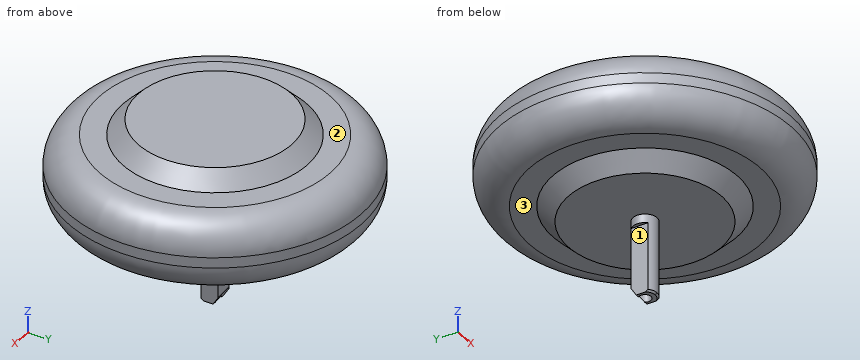
from build123d import *

# Parameters (mm, degrees)
SKETCH_1_R           = 85
EXTRUDE_1_DEPTH      = 21
SKETCH_2_R           = 54.5
EXTRUDE_2_DEPTH      = 30
CHAMFER_1_SIZE       = 10
SKETCH_3_R           = 7
EXTRUDE_3_DEPTH      = 45
SKETCH_5_OUTSIDE_W   = 224.47
SKETCH_5_OUTSIDE_H   = 224.47
SKETCH_5_OUTSIDE_W_2 = 9.85
SKETCH_5_OUTSIDE_H_2 = 14
CUT_EXTRUDE_1_DEPTH  = 40
CHAMFER_3_SIZE       = 1
SKETCH_7_R           = 3.5
CUT_EXTRUDE_2_DEPTH  = 45
FILLET_1_R           = 18
CUT_EXTRUDE_3_REACH  = 146.695


with BuildPart() as part:
    # 草图1 → 凸台-拉伸1 (new, symmetric)
    with BuildSketch(Plane.XY):
        with Locations(Location((0, 0, 0), (0, 0, 180))):
            Circle(SKETCH_1_R)
    extrude(amount=EXTRUDE_1_DEPTH, both=True)

    # 草图2 → 凸台-拉伸2 (add, symmetric)
    with BuildSketch(Plane.XY):
        Circle(SKETCH_2_R)
    extrude(amount=EXTRUDE_2_DEPTH, both=True)

    # 倒角1
    # the kernel refuses this chamfer: 10 mm, written as the material it takes off along each edge
    with BuildSketch(Plane(origin=(0, 0, -30), x_dir=(1, 0, 0), z_dir=(0, -1, 0))) as chamfer_1_piece_1_section:
        Polygon((54.5, CHAMFER_1_SIZE), (54.5 - CHAMFER_1_SIZE, 0), (54.5, 0), align=None)
    chamfer_1_piece_1 = revolve(axis=Axis((0, 0, -30), (0, 0, 1)), mode=Mode.PRIVATE)
    chamfer_1_piece_1 = split(chamfer_1_piece_1, bisect_by=Plane(origin=(-49.041649133, 0, -21), z_dir=(0, 0, -1)), keep=Keep.TOP, mode=Mode.PRIVATE)
    add(chamfer_1_piece_1, mode=Mode.SUBTRACT)
    with BuildSketch(Plane(origin=(0, 0, 30), x_dir=(1, 0, 0), z_dir=(0, -1, 0))) as chamfer_1_piece_2_section:
        Polygon((54.5, -CHAMFER_1_SIZE), (54.5 - CHAMFER_1_SIZE, 0), (54.5, 0), align=None)
    chamfer_1_piece_2 = revolve(axis=Axis((0, 0, 30), (0, 0, 1)), mode=Mode.PRIVATE)
    chamfer_1_piece_2 = split(chamfer_1_piece_2, bisect_by=Plane(origin=(-49.041649133, 0, 21), z_dir=(0, 0, 1)), keep=Keep.TOP, mode=Mode.PRIVATE)
    add(chamfer_1_piece_2, mode=Mode.SUBTRACT)

    # 草图3 → 凸台-拉伸3 (add)
    with BuildSketch(Plane(origin=(0, 0, -30), x_dir=(-1, 0, 0), z_dir=(0, 0, -1))):
        with Locations(Location((0, 0, 0), (0, 0, 180))):
            Circle(SKETCH_3_R)
    extrude(amount=EXTRUDE_3_DEPTH)

    # 草图5 outside → 切除-拉伸1 (cut)
    with BuildSketch(Plane(origin=(0, 0, -75), x_dir=(-1, 0, 0), z_dir=(0, 0, -1))):
        Rectangle(SKETCH_5_OUTSIDE_W, SKETCH_5_OUTSIDE_H)
        Rectangle(SKETCH_5_OUTSIDE_W_2, SKETCH_5_OUTSIDE_H_2, mode=Mode.SUBTRACT)
    extrude(amount=-CUT_EXTRUDE_1_DEPTH, mode=Mode.SUBTRACT)

    # 倒角3
    # the kernel refuses this chamfer: 1 mm, written as the material it takes off along each edge
    with BuildSketch(Plane(origin=(0, 0, -75), x_dir=(-0.9118755958915212, 0.4104666827130834, 0), z_dir=(-0.4104666827130834, -0.9118755958915212, 0))) as chamfer_3_piece_1:
        Polygon((7, -CHAMFER_3_SIZE), (7 - CHAMFER_3_SIZE, 0), (7, 0), align=None)
    revolve(axis=Axis((0, 0, -75), (0, 0, -1)), revolution_arc=65.76584555, mode=Mode.SUBTRACT)
    with BuildSketch(Plane(origin=(0, 0, -75), x_dir=(0.9118755958915, -0.41046668271313064, 0), z_dir=(0.41046668271313064, 0.9118755958915, 0))) as chamfer_3_piece_2:
        Polygon((7, -CHAMFER_3_SIZE), (7 - CHAMFER_3_SIZE, 0), (7, 0), align=None)
    revolve(axis=Axis((0, 0, -75), (0, 0, -1)), revolution_arc=65.76584555, mode=Mode.SUBTRACT)
    with BuildSketch(Plane(origin=(0, 0, -75), x_dir=(0, -1, 0), z_dir=(1, 0, 0))) as chamfer_3_piece_3:
        Polygon((7, -CHAMFER_3_SIZE), (7 - CHAMFER_3_SIZE, 0), (7, 0), align=None)
    revolve(axis=Axis((0, 0, -75), (0, 0, -1)), revolution_arc=65.76584555, mode=Mode.SUBTRACT)
    with BuildSketch(Plane(origin=(0, 0, -75), x_dir=(0, 1, 0), z_dir=(-1, 0, 0))) as chamfer_3_piece_4:
        Polygon((7, -CHAMFER_3_SIZE), (7 - CHAMFER_3_SIZE, 0), (7, 0), align=None)
    revolve(axis=Axis((0, 0, -75), (0, 0, -1)), revolution_arc=65.76584555, mode=Mode.SUBTRACT)

    # 草图7 → 切除-拉伸2 (cut)
    with BuildSketch(Plane(origin=(0, 0, -75), x_dir=(-1, 0, 0), z_dir=(0, 0, -1))):
        Circle(SKETCH_7_R)
    extrude(amount=-CUT_EXTRUDE_2_DEPTH, mode=Mode.SUBTRACT)

    # 圆角1
    fillet_1_edges = [part.edges().sort_by_distance(p)[0] for p in [
        (85, 0, -21),
        (85, 0, 21),
    ]]
    fillet(fillet_1_edges, radius=FILLET_1_R)

    # 草图8 → 切除-拉伸3 (cut, up to next)
    with BuildSketch(Plane(origin=(4.925, 0, 0), x_dir=(0, 0, -1), z_dir=(1, 0, 0)), mode=Mode.PRIVATE) as cut_extrude_3_sk1:
        Polygon((75, 2), (75, 7), (67, 7), align=None)
    cut_extrude_3_tool1 = extrude(cut_extrude_3_sk1.sketch, amount=-CUT_EXTRUDE_3_REACH, mode=Mode.PRIVATE) & part.part
    add(cut_extrude_3_tool1.solids().sort_by_distance((4.925, 5.333333, -72.333333))[0], mode=Mode.SUBTRACT)


solid = part.part
Source: CAD feature listing. Evaluate the final solid. Frame: model axes, mm. Face numbers are marked on the shaded views. A direction names the side the tool comes from. Coordinates: 2 decimals unless noted, no trailing zeros. Write each loop counter-clockwise with the first axis right and the second up, starting at its lowest first coordinate (ties: lowest second). Pieces come first, ordered by that corner, then holes. Notation, with made-up numbers: M 32,-13.75 L 82,-13.75 A28 cw 82,4.25 Z; hole C 84.25,-17.75 d4. An arc over 180 degrees is marked long. Use a Markdown table: item, result.
1) First-contact query: pin 1 Ø2 at (x, y) = (-27, -18.5) entering from -Z; pin 2 Ø5 at (x, z) = (-66.5, -4) entering from -Y; pin 3 Ø1.7 at (x, y) = (-6, -1) entering from -Z. Flat tips, straight axial feed; report the tip coordinate or a pass-through.
Conclusion:
| item | result |
|---|---|
| pin 1 | stops at z = -30 |
| pin 2 | stops at y = -55.9 |
| pin 3 | stops at z = -35 |
2) Section C-C, the plane z = 11. Output: boundary loops of the cut face in (x, y), then the cut area to 3 significant figures.
Conclusion:
| item | result |
|---|---|
| outline | C 0,0 d166.25 |
| area | 21,700 mm^2 |
3) Reachability of the marked faces 1, 2 and 3 from +Z, -Z, +X, -X, +Y, -Y: full face, straight path, thin tool, end or side. Return the list, or none.
Conclusion:
| item | result |
|---|---|
| face 1 | -Z, -X, +Y, -Y |
| face 2 | +Z |
| face 3 | -Z |
4) Ray query, L1, parallel to Y at x = 0, z = -63; L2, parallel to X at y = 0, z = -59 (3 decimals); L3, parallel to Z at x = -60, y = -17. Return the intervals inside material, ascending.
Conclusion:
| item | result |
|---|---|
| L1 | y = -7 to -3.5, 3.5 to 7 |
| L2 | x = -4.925 to -3.5, 3.5 to 4.925 |
| L3 | z = -21 to 21 |
5) Section B-B, the plane z = -0.5. Output: boundary loops of the cut face in (x, y).
Conclusion:
| item | result |
|---|---|
| outline | C 0,0 d170 |
6) Section A-A, the plane z = -61. Output: boundary loops of the cut face in (x, y) (3 decimals).
Conclusion:
| item | result |
|---|---|
| outline | M -4.925,-4.974 A7 ccw 4.925,-4.974 L 4.925,4.974 A7 ccw -4.925,4.974 Z; hole C 0,0 d7 |
